Autodesk Inventor part; units mm, degrees
ref_plane "Work Plane2" through (0, 3.5617, 0) normal (0, -1, 0) x (1, 0, 0)
ref_plane "YZ Plane" through (0, 0, 0) normal (1, 0, 0) x (0, 1, 0)
ref_plane "XZ Plane" through (0, 0, 0) normal (0, 1, 0) x (-1, 0, 0)
sketch "Sketch1" plane through (0, 0, 0) normal (0, 1, 0) x (-1, 0, 0)
  circle A0 centre (0, 0) radius 4
  dimension "d0" = 8
extrude "Extrusion1" add sketch "Sketch1" against normal mid plane 18
sketch "Sketch2" plane through (0, -9, 0) normal (0, -1, 0) x (1, 0, 0)
  circle A0 centre (0, 0) radius 4
  line L0 (-5.6, 0) -> (5.6, 0)
  line L1 (-1.5, -1.5) -> (1.5, -1.5)
  line L2 (1.5, -1.5) -> (1.5, 1.5)
  line L3 (1.5, 1.5) -> (-1.5, 1.5)
  line L4 (-1.5, 1.5) -> (-1.5, -1.5)
  dimension "d3" = 3
  dimension "d4" = 3
  dimension "d5" = 1.5
  dimension "d6" = 1.5
extrude "Extrusion2" add sketch "Sketch2" along normal blind 4 contours L2 L1 L4 L0 | L0 L4 L3 L2
fillet "Fillet1" radius 0.2 8 edges at (1.5, -11, 1.5) (-1.5, -11, 1.5) (1.5, -11, -1.5) (0, -13, -1.5) (-1.5, -13, 0) (0, -13, 1.5) (1.5, -13, 0) (-1.5, -11, -1.5)
sketch "Sketch3" plane through (0, 0, 0) normal (0, 0, 1) x (1, 0, 0)
  line L0 (0, -4.8) -> (0, 0)
  line L1 (2.8, 0) -> (2.8, -4.8)
  arc A0 (-0.35, -2.4) -> (3.15, -2.4) centre (1.4, -2.4) ccw
  line L2 (0, -2.4) -> (2.8, -2.4) construction
  line L3 (-4, -9) -> (-4, 9)
  line L4 (-4, 9) -> (4, 9)
  line L5 (4, 9) -> (4, -9)
  line L6 (4, -9) -> (1.5, -9)
  line L7 (1.5, -9) -> (1.5, -12.8)
  arc A1 (1.3, -13) -> (1.5, -12.8) centre (1.3, -12.8) ccw
  line L8 (1.3, -13) -> (-1.3, -13)
  arc A2 (-1.5, -12.8) -> (-1.3, -13) centre (-1.3, -12.8) ccw
  line L9 (-1.5, -12.8) -> (-1.5, -9)
  line L10 (-1.5, -9) -> (-4, -9)
  line L11 (-1.5, -10.9) -> (1.5, -10.9) construction
  arc A3 (-1.75, -10.9) -> (1.75, -10.9) centre (0, -10.9) ccw
  line L12 (1.5, -10.9) -> (2.2631, -10.9) construction
  line L13 (-1.5, -10.9) -> (-1.9787, -10.9) construction
  line L14 (-1.75, -10.9) -> (1.75, -10.9)
  point P0 (1.4, -2.4)
  dimension "d10" = 1.75
  dimension "d11" = 3.5
revolve "Revolution1" add sketch "Sketch3" angle 360 about axis through (1.5, -10.9, 0) along (1, 0, 0) contours L14 L7 A3 L9 | L9 A3 L14 | L14 A3 L7
mirror "Mirror1" about plane through (0, 0, 0) normal (0, 1, 0) of "Extrusion2", "Revolution1", "Fillet1"
chamfer "Chamfer2" distance 0.3 angle 45 2 edges at (4, -9, 0) (4, 9, 0)
ref_plane "Work Plane2" through (0, 3.5617, 0) normal (0, -1, 0) x (1, 0, 0)
split_face "Split2"
equation "\"d3\" = d4"
equation "\"d5\" = 0.5 * d4"
equation "\"d6\" = 0.5 * d4"
properties part number "473-01" material "Steel"
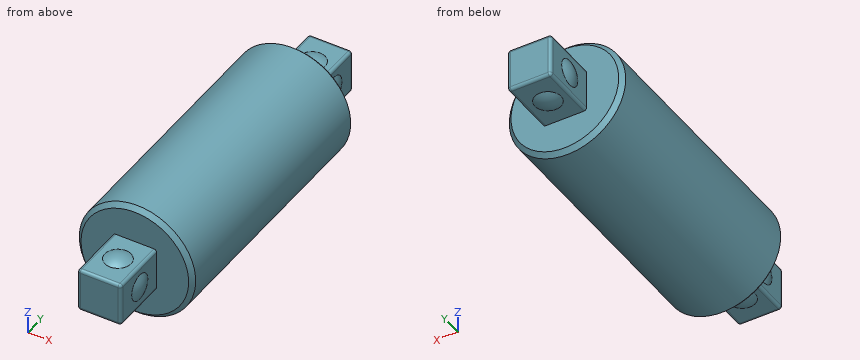
Can you work these out from the model? Positions are in its coordinate system, mm. Round coordinates to 2 decimals unless told otherwise and drop trailing zeros. Loops run counter-clockwise (first coordinate to the right, second up) from the corner with the lowest first, then second, coordinate; pieces in that order, holes last. Notation, with made-up numbers: (11, 79.5) - (48, 79.5) arc R21 cw to (48, 115.5) - close; hole circle Ø9 at (37, 8.5). An arc over 180 degrees is marked (long way). Answer in a Markdown table with one row per item. Add a question column.
Q1. I want a section at C-C on y = -5.75. List the corners of the cut face in (x, z) for me.
Q2. I want a section at B-B on z = 0. List the corners of the cut face in (x, y) for me, and give its area (3 significant figures).
Q3. I need wall thicknesses on L1, parallel to Z at x = 0.75, y = -9.25; L2, parallel to Y at x = -2.5, z = 0.5; L3, parallel to X at y = -6.5, z = -1. Which ranges of each line are inside material? Lowest first, please.
Q4. I want a section at A-A on x = 0. List the corners of the cut face in (y, z) for me, and give its area (3 significant figures).
Q5. For pin 1 Ø1 at (x, y) = (3, -5.5) entering from +Z; pin 2 Ø1.3 at (x, y) = (0.5, 10.5) entering from +Z; pin 3 Ø2 at (x, y) = (0, -10.5) entering from -Z, each with a flat end and sliding along its axis, tell me the tip position at first contact or that it passes through.
A:
| question | item | result |
|---|---|---|
| 1 | outline | circle Ø8 at (0, 0) |
| 2 | outline | (-4, -8.7) - (-3.7, -9) - (-1.5, -9) - (-1.5, -10) arc R1.75 ccw to (-1.5, -11.8) - (-1.5, -12.8) arc R0.2 ccw to (-1.3, -13) - (1.3, -13) arc R0.2 ccw to (1.5, -12.8) - (1.5, -11.8) arc R1.75 ccw to (1.5, -10) - (1.5, -9) - (3.7, -9) - (4, -8.7) - (4, 8.7) - (3.7, 9) - (1.5, 9) - (1.5, 10) arc R1.75 ccw to (1.5, 11.8) - (1.5, 12.8) arc R0.2 ccw to (1.3, 13) - (-1.3, 13) arc R0.2 ccw to (-1.5, 12.8) - (-1.5, 11.8) arc R1.75 ccw to (-1.5, 10) - (-1.5, 9) - (-3.7, 9) - (-4, 8.7) - close |
| 2 | area | 169 mm^2 |
| 3 | L1 | -1.5 to 1.5 |
| 3 | L2 | -9 to 9 |
| 3 | L3 | -3.87 to 3.87 |
| 4 | outline | (-13, -1.3) arc R0.2 ccw to (-12.8, -1.5) - (-11.8, -1.5) arc R1.75 ccw to (-10, -1.5) - (-9, -1.5) - (-9, -3.7) - (-8.7, -4) - (8.7, -4) - (9, -3.7) - (9, -1.5) - (10, -1.5) arc R1.75 ccw to (11.8, -1.5) - (12.8, -1.5) arc R0.2 ccw to (13, -1.3) - (13, 1.3) arc R0.2 ccw to (12.8, 1.5) - (11.8, 1.5) arc R1.75 ccw to (10, 1.5) - (9, 1.5) - (9, 3.7) - (8.7, 4) - (-8.7, 4) - (-9, 3.7) - (-9, 1.5) - (-10, 1.5) arc R1.75 ccw to (-11.8, 1.5) - (-12.8, 1.5) arc R0.2 ccw to (-13, 1.3) - close |
| 4 | area | 169 mm^2 |
| 5 | pin 1 | z = 3.12 |
| 5 | pin 2 | z = 1.75 |
| 5 | pin 3 | z = -1.75 |
